from build123d import *

# Parameters (mm, degrees)
SKETCH1_W           = 45
SKETCH1_H           = 25
SKETCH1_R           = 2.225
BOSS_EXTRUDE1_DEPTH = 74
SKETCH2_R           = 4.5
SKETCH2_R_2         = 2.725
CUT_EXTRUDE1_DEPTH  = 82.284992465
SKETCH3_W           = 45
SKETCH3_H           = 12
CUT_EXTRUDE2_DEPTH  = 60
FILLET4_R           = 20
SKETCH4_R           = 3.725
CUT_EXTRUDE4_DEPTH  = 27
FILLET5_R           = 20
FILLET6_R           = 2


with BuildPart() as part:
    # Sketch1 → Boss-Extrude1 (new body)
    with BuildSketch(Plane.XY):
        Rectangle(SKETCH1_W, SKETCH1_H)
        with Locations((-8.25, 6)):
            Circle(SKETCH1_R, mode=Mode.SUBTRACT)
        with Locations((8.25, 6)):
            Circle(SKETCH1_R, mode=Mode.SUBTRACT)
    extrude(amount=BOSS_EXTRUDE1_DEPTH)

    # Sketch2 → Cut-Extrude1 (cut, through all)
    with BuildSketch(Plane.XZ.offset(12.5)):
        with Locations(Location((0, 50, 0), (0, 0, 270))):
            Circle(SKETCH2_R)
        with Locations(Location((-16.5, 50, 0), (0, 0, 270))):
            Circle(SKETCH2_R_2)
        with Locations(Location((16.5, 50, 0), (0, 0, 270))):
            Circle(SKETCH2_R_2)
    extrude(amount=-CUT_EXTRUDE1_DEPTH, mode=Mode.SUBTRACT)

    # Sketch3 → Cut-Extrude2 (cut)
    with BuildSketch(Plane.XY.offset(74)):
        with Locations((0, 6.5)):
            Rectangle(SKETCH3_W, SKETCH3_H)
    extrude(amount=-CUT_EXTRUDE2_DEPTH, mode=Mode.SUBTRACT)

    # Fillet4
    # the kernel refuses this fillet: 20 mm, written as the material it adds along each edge
    with BuildSketch(Plane(origin=(22.5, 0.5, 14), x_dir=(0, 1, 0), z_dir=(-1, 0, 0))) as fillet4_piece_1_section:
        with BuildLine():
            CenterArc((20, -18.33030278), FILLET4_R, 113.578178478, 66.421821522)
            Line((0, -18.33030278), (-0.4, -18.33030278))
            Line((-0.4, -18.33030278), (-0.4, 0))
            Line((-0.4, 0), (0, 0.4))
            ThreePointArc((0, 0.4), (6, 0.4), (11.84, 0.366606056))
            Line((11.84, 0.366606056), (12, 0))
        make_face()
    fillet4_piece_1 = extrude(amount=45, mode=Mode.PRIVATE)
    fillet4_piece_1 = fillet4_piece_1 - Plane(origin=(8.25, 6, 18.573304712), x_dir=(1, 0, 0), z_dir=(0, 0, -1)) * Cylinder(2.225, 164, mode=Mode.PRIVATE)
    fillet4_piece_1 = fillet4_piece_1 - Plane(origin=(-8.25, 6, 18.573304712), x_dir=(1, 0, 0), z_dir=(0, 0, -1)) * Cylinder(2.225, 164, mode=Mode.PRIVATE)
    add(fillet4_piece_1)

    # Sketch4 → Cut-Extrude4 (cut)
    with BuildSketch(Plane.XY.offset(14)):
        with Locations(Location((-8.25, 6, 0), (0, 0, 180))):
            Circle(SKETCH4_R)
        with Locations(Location((8.25, 6, 0), (0, 0, 180))):
            Circle(SKETCH4_R)
    extrude(amount=CUT_EXTRUDE4_DEPTH, mode=Mode.SUBTRACT)

    # Fillet5
    fillet5_edges = [part.edges().sort_by_distance(p)[0] for p in [
        (-22.5, -6, 74),
        (22.5, -6, 74),
    ]]
    fillet(fillet5_edges, radius=FILLET5_R)

    # Fillet6
    fillet6_edges = [part.edges().sort_by_distance(p)[0] for p in [
        (-22.5, 12.5, 7),
        (22.5, 12.5, 7),
        (22.5, 0.5, 43.16515139),
        (-22.5, 0.5, 43.16515139),
        (22.5, 3.766799469, 21.37585163),
        (-22.5, 3.766799469, 21.37585163),
        (0, 0.5, 74),
        (0, -12.5, 74),
        (-16.642135624, 0.5, 68.142135624),
        (16.642135624, 0.5, 68.142135624),
        (22.5, -12.5, 27),
        (-22.5, -12.5, 27),
        (-16.642135624, -12.5, 68.142135624),
        (16.642135624, -12.5, 68.142135624),
    ]]
    fillet(fillet6_edges, radius=FILLET6_R)


solid = part.part
The model under review builds one solid part; all positions refer to its coordinate system, in mm. A direction names the side the tool comes from. Coordinates: 2 decimals unless noted, no trailing zeros. Write each loop counter-clockwise with the first axis right and the second up, starting at its lowest first coordinate (ties: lowest second). Pieces come first, ordered by that corner, then holes. Notation, with made-up numbers: (20.5, -2.75) -> (30.5, -2.75) arc R26 cw to (30.5, 29.25) -> close; hole circle Ø8 at (88, 41). An arc over 180 degrees is marked (long way). Answer in a Markdown table with one row per item.
1. For faces 4 (the flat face through (-5, 0.5, 52)), 5 (the flat face through (-10, 8, 14)), 6 (the cylindrical face through (-21.9, -11.93, 27.38)), 7 (the cylindrical face through (-21.93, -0.1, 43.32)), list the 3-axis set-ups (+Z, -Z, +X, -X, +Y, -Y) from which the entire face can be reached by the end or side of a thin tool; tool diameter is ignored.
Answers below:
| item | result |
|---|---|
| face 4 | +Z, +X, -X, +Y |
| face 5 | +Z |
| face 6 | +Z, -Z, -X, -Y |
| face 7 | +Z, -X, +Y |
2. Clearance check with a flat-ended pin moving along its axis: pin 1 Ø8.5 at (x, z) = (-16.5, 50) entering from +Y. State where the tip first meets the part, or that it passes through.
Answers below:
| item | result |
|---|---|
| pin 1 | stops at y = 0.5 |
3. We need section A-A, the plane z = 50. State the section outline as (x, y) points (3 decimals).
Answers below:
| item | result |
|---|---|
| outline | (-22.5, -10.5) arc R2 ccw to (-20.5, -12.5) -> (-19.225, -12.5) -> (-19.225, 0.5) -> (-20.5, 0.5) arc R2 ccw to (-22.5, -1.5) -> close; (-13.775, -12.5) -> (-4.5, -12.5) -> (-4.5, 0.5) -> (-13.775, 0.5) -> close; (4.5, -12.5) -> (13.775, -12.5) -> (13.775, 0.5) -> (4.5, 0.5) -> close; (19.225, -12.5) -> (20.5, -12.5) arc R2 ccw to (22.5, -10.5) -> (22.5, -1.5) arc R2 ccw to (20.5, 0.5) -> (19.225, 0.5) -> close |
4. Wall thickness on probe 1 along X at (y, z) = (6, 10) (3 decimals); probe 2 along X at (y, z) = (5.5, 15.5); probe 3 along Y at (x, z) = (17.5, 56): over which ranges is each line inside the solid? List them lowest first. Write a range as [from, to].
Answers below:
| item | result |
|---|---|
| probe 1 | x = [-22.5, -10.475], [-6.025, 6.025], [10.475, 22.5] |
| probe 2 | x = [-22.5, -11.94], [-4.56, 4.56], [11.94, 22.5] |
| probe 3 | y = [-12.5, 0.5] |
5. We need section B-B, the plane y = 4.75. Give the number of separate pieces and of enclosed holes in the cut face, and give its area (3 significant figures).
Answers below:
| item | result |
|---|---|
| separate pieces | 3 |
| enclosed holes | 0 |
| area | 710 mm^2 |
6. Draft analysis for pull direction Y (two halves, no side actions). For faces 1 (the flat face through (0, -12.5, 35)), 2 (the cylindrical face through (8.735, 2.307, 17.854)), 3 (the flat face through (0, -6, 74)), state which applies: +Y half, -Y half, draft (parallel to the pull), parting line (faces both ways), or undercut.
Answers below:
| item | result |
|---|---|
| face 1 | -Y half |
| face 2 | undercut |
| face 3 | draft |
